Verification items for the finished model (mm, model axes). A direction names the side the tool comes from. Give positions to 0.01 mm unless a question says otherwise; leave off trailing zeros. Order: outer loops, then holes, each group sorted by start corner. A loop starts at its lowest first (then second) coordinate and runs counter-clockwise, first axis right, second up. Notation, with made-up numbers: (78.5, 19) -> (91.5, 19) arc R12 cw to (91.5, 23) -> close; hole circle Ø7 at (35, -20). An arc over 180 degrees is marked (long way). Return JSON: item names as keys, results as strings. Group by question number.
(1) Cross-section at A-A on z = 26.25. Enter the section's corners in (x, y) (3 decimals).
(2) Cross-section at C-C on y = -24.5. Enter the section's corners in (x, z), then the cut area to 3 significant figures.
(3) Cross-section at D-D on x = -14.5. Enter the section's corners in (y, z) (3 decimals), then the cut area to 3 significant figures.
(4) Thickness scan on line 1 along X through (y, z) = (-40, 26); line 2 along Z through (x, y) = (-41, 35); line 3 along Y through (x, z) = (-17.5, 13) (3 decimals). Record the ranges inside material, lowest first.
(5) Cross-section at B-B on x = -32. State how many separate pieces and enclosed holes the cut face has, then the cut area to 3 significant figures.
(6) Depth check by flat-ended pin: pin 1 Ø4 at (x, y) = (62, 3) entering from +Z; pin 2 Ø4.5 at (x, y) = (-31.5, -36) entering from +Z; pin 3 Ø6.5 at (x, z) = (-38.01, 32.26) entering from -Y (3 decimals); pin 4 Ø12 at (x, y) = (-41.5, -11) entering from +Z. Enter the tip coordinate at first touch or a pass-through.
(7) Tool access check on faces 3 (the face through (-3, -36, 13.75)), 4 (the face through (33.382, 13.474, 1.479)), 5 (the face through (63, 0, 8.875)), 6 (the face through (-3, 36.575, 7)), 7 (the face through (-23.934, -40.86, 24.298)). Record the directions out of +Z, -Z, +X, -X, +Y, -Y that give a thin tool (end or side, any length) a straight path to the whole face; none if there is none.
(8) Release check for a two-part mould opening along X. For faces 1 (the face through (33.908, -40.86, 18.351)), 2 (the face through (-1, -2, 0)) record: pulls with the +X half, pulls with the -X half, needs draft (parallel to the pull), parting line crosses it, or undercut.
from build123d import *

# Parameters (mm, degrees)
SKETCH1_W           = 130
SKETCH1_H           = 5
BOSS_EXTRUDE1_DEPTH = 38.75
BOSS_EXTRUDE2_DEPTH = 3
SKETCH1_5_W         = 125
SKETCH1_5_H         = 1.75
BOSS_EXTRUDE3_DEPTH = 11.75
BOSS_EXTRUDE5_START = 11.75
SKETCH1_7_W         = 125
SKETCH1_7_H         = 4.3
BOSS_EXTRUDE5_DEPTH = 2
SKETCH2_R           = 2
SKETCH2_R_2         = 4.124206023
CUT_EXTRUDE1_DEPTH  = 13.75
SKETCH1_9_W         = 5
SKETCH1_9_H         = 2.55
SKETCH1_9_H_2       = 1.75
BOSS_EXTRUDE7_DEPTH = 10
SKETCH3_W           = 7.75
SKETCH3_H           = 10
CUT_EXTRUDE2_DEPTH  = 10


with BuildPart() as part:
    # Sketch1 → Boss-Extrude1 (new body)
    with BuildSketch(Plane.XY):
        with Locations((0, -40.825)):
            Rectangle(SKETCH1_W, SKETCH1_H)
    extrude(amount=BOSS_EXTRUDE1_DEPTH)

    # Sketch1_5 → Boss-Extrude3 (add)
    with BuildSketch(Plane.XY):
        with Locations((-2.5, 37.45)):
            Rectangle(SKETCH1_5_W, SKETCH1_5_H)
        with Locations((-2.5, -37.45)):
            Rectangle(SKETCH1_5_W, SKETCH1_5_H)
    extrude(amount=BOSS_EXTRUDE3_DEPTH)


with BuildPart() as body_2:
    # Sketch1_4 → Boss-Extrude2 (new body)
    with BuildSketch(Plane.XY):
        Polygon((60, -27.329770154), (7.5, 0), (60, 27.329770154), (60, 36.575), (-65, 36.575), (-65, -36.575), (60, -36.575), align=None)
        Polygon((-60, 27.329770154), (-7.5, 0), (-60, -27.329770154), align=None, mode=Mode.SUBTRACT)
        Polygon((0, -7.5), (48.024553174, -32.5), (-48.024553174, -32.5), align=None, mode=Mode.SUBTRACT)
        Polygon((48.024553174, 32.5), (0, 7.5), (-48.024553174, 32.5), align=None, mode=Mode.SUBTRACT)
    extrude(amount=BOSS_EXTRUDE2_DEPTH)



with BuildPart() as boss_extrude3_piece_1:
    # of the separate pieces the step leaves, piece 1, a body of its own (boss_extrude3_pieces)
    add(part.part.solids().sort_by_distance((-65, -43.325, 0))[0])



with BuildPart() as boss_extrude3_piece_2:
    # of the separate pieces the step leaves, piece 2, a body of its own (boss_extrude3_pieces)
    add(part.part.solids().sort_by_distance((60, 36.575, 0))[0])


with BuildPart() as boss_extrude3_piece_1_1:
    add(boss_extrude3_piece_1.part)

    add(boss_extrude3_piece_2.part)  # Boss-Extrude5 merges Boss-Extrude3 piece 2
    # Sketch1_7 → Boss-Extrude5 (add)
    with BuildSketch(Plane.XY.offset(BOSS_EXTRUDE5_START)):
        with Locations((-2.5, 36.175)):
            Rectangle(SKETCH1_7_W, SKETCH1_7_H)
        with Locations((-2.5, -36.175)):
            Rectangle(SKETCH1_7_W, SKETCH1_7_H)
    extrude(amount=BOSS_EXTRUDE5_DEPTH)

    # Sketch2 → Cut-Extrude1 (cut)
    with BuildSketch(Plane.XZ.offset(43.325)):
        with Locations((32, 34.75)):
            Circle(SKETCH2_R)
        with Locations((23.5, 26.25)):
            Circle(SKETCH2_R)
        with Locations((0, 34.75)):
            Circle(SKETCH2_R)
        with Locations(Location((0, 17.75, 0), (0, 0, 90))):
            Circle(SKETCH2_R)
        with Locations((0, 26.25)):
            Circle(SKETCH2_R_2)
        with Locations((38.01040764, 32.26040764)):
            Circle(SKETCH2_R)
        with Locations((40.5, 26.25)):
            Circle(SKETCH2_R)
        with Locations((38.01040764, 20.23959236)):
            Circle(SKETCH2_R)
        with Locations((32, 17.75)):
            Circle(SKETCH2_R)
        with Locations((25.98959236, 20.23959236)):
            Circle(SKETCH2_R)
        with Locations((25.98959236, 32.26040764)):
            Circle(SKETCH2_R)
        with Locations((-38.01040764, 20.23959236)):
            Circle(SKETCH2_R)
        with Locations((-32, 17.75)):
            Circle(SKETCH2_R)
        with Locations((-25.98959236, 20.23959236)):
            Circle(SKETCH2_R)
        with Locations((-23.5, 26.25)):
            Circle(SKETCH2_R)
        with Locations((-25.98959236, 32.26040764)):
            Circle(SKETCH2_R)
        with Locations((-32, 34.75)):
            Circle(SKETCH2_R)
        with Locations((-38.01040764, 32.26040764)):
            Circle(SKETCH2_R)
        with Locations((-40.5, 26.25)):
            Circle(SKETCH2_R)
    extrude(amount=-CUT_EXTRUDE1_DEPTH, mode=Mode.SUBTRACT)


with BuildPart() as body_2_1:
    add(body_2.part)

    add(boss_extrude3_piece_1_1.part)  # Boss-Extrude7 merges Boss-Extrude3 piece 1
    # Sketch1_9 → Boss-Extrude7 (add)
    with BuildSketch(Plane.XY):
        Polygon((65, -34.025), (65, 34.025), (60, 34.025), (60, 32.5), (60, 27.329770154), (60, -27.329770154), (60, -32.5), (60, -34.025), align=None)
        with Locations((62.5, -35.3)):
            Rectangle(SKETCH1_9_W, SKETCH1_9_H)
        with Locations((62.5, -37.45)):
            Rectangle(SKETCH1_9_W, SKETCH1_9_H_2)
        with Locations((62.5, 35.3)):
            Rectangle(SKETCH1_9_W, SKETCH1_9_H)
        with Locations((62.5, 37.45)):
            Rectangle(SKETCH1_9_W, SKETCH1_9_H_2)
    extrude(amount=BOSS_EXTRUDE7_DEPTH)

    # Sketch3 → Cut-Extrude2 (cut)
    with BuildSketch(Plane(origin=(65, 0, 0), x_dir=(0, 0, -1), z_dir=(1, 0, 0))):
        with Locations((-5, 5)):
            Rectangle(SKETCH3_W, SKETCH3_H)
        with Locations((-5, -5)):
            Rectangle(SKETCH3_W, SKETCH3_H)
    extrude(amount=-CUT_EXTRUDE2_DEPTH, mode=Mode.SUBTRACT)


solid = body_2_1.part
Verdict:
{
 "1": {"outline": "(-65, -43.325) -> (-42.5, -43.325) -> (-42.5, -38.325) -> (-65, -38.325) -> close; (-38.5, -43.325) -> (-25.5, -43.325) -> (-25.5, -38.325) -> (-38.5, -38.325) -> close; (-21.5, -43.325) -> (-4.124, -43.325) -> (-4.124, -38.325) -> (-21.5, -38.325) -> close; (4.124, -43.325) -> (21.5, -43.325) -> (21.5, -38.325) -> (4.124, -38.325) -> close; (25.5, -43.325) -> (38.5, -43.325) -> (38.5, -38.325) -> (25.5, -38.325) -> close; (42.5, -43.325) -> (65, -43.325) -> (65, -38.325) -> (42.5, -38.325) -> close"},
 "2": {"outline": "(-65, 0) -> (-60, 0) -> (-60, 3) -> (-65, 3) -> close; (-54.56, 0) -> (-32.66, 0) -> (-32.66, 3) -> (-54.56, 3) -> close; (32.66, 0) -> (54.56, 0) -> (54.56, 3) -> (32.66, 3) -> close; (60, 0) -> (65, 0) -> (65, 10) -> (60, 10) -> close", "area": "196 mm²"},
 "3": {"outline": "(-43.325, 0) -> (-32.5, 0) -> (-32.5, 3) -> (-36.575, 3) -> (-36.575, 11.75) -> (-34.025, 11.75) -> (-34.025, 13.75) -> (-38.325, 13.75) -> (-38.325, 38.75) -> (-43.325, 38.75) -> close; (-15.048, 0) -> (-3.644, 0) -> (-3.644, 3) -> (-15.048, 3) -> close; (3.644, 0) -> (15.048, 0) -> (15.048, 3) -> (3.644, 3) -> close; (32.5, 0) -> (38.325, 0) -> (38.325, 13.75) -> (34.025, 13.75) -> (34.025, 11.75) -> (36.575, 11.75) -> (36.575, 3) -> (32.5, 3) -> close", "area": "345 mm²"},
 "4": {"line 1": "-65 to -42.48, -38.52 to -25.48, -21.52 to -4.12, 4.12 to 21.52, 25.48 to 38.52, 42.48 to 65", "line 2": "0 to 3, 11.75 to 13.75", "line 3": "-43.325 to -34.025, 34.025 to 38.325"},
 "5": {"separate pieces": "6", "enclosed holes": "0", "area": "305 mm²"},
 "6": {"pin 1": "z = 10", "pin 2": "z = 13.75", "pin 3": "y = -43.325", "pin 4": "z = 3"},
 "7": {"face 3": "+Z, +X, -X, +Y", "face 4": "+Z, -Z", "face 5": "+X, -X", "face 6": "-X", "face 7": "+Y, -Y"},
 "8": {"face 1": "undercut", "face 2": "needs draft"}
}
